```python
from build123d import *

# Parameters (mm, degrees)
F1_DEPTH  = 2
F2_DEPTH  = 25
F3_T      = -2
F4_W      = 8
F4_H      = 8
F5_DEPTH  = 25
F6_W      = 35
F6_H      = 11.5
F6_R      = 1.1
F7_DEPTH  = 30
F8_DEPTH  = 10
F9_W      = 25
F9_H      = 11.5
F10_DEPTH = 25
F11_DEPTH = 10


# Not quite as in the source:
# - a feature names something its author has since deleted; it is built from what else it names


with BuildPart() as f1:
    # F0 (on Top) → F1 (new body)
    with BuildSketch(Plane.XY):
        with BuildLine():
            Line((-20, -62.5), (20, -62.5))
            ThreePointArc((20, -62.5), (34.1421356237, -56.6421356237), (40, -42.5))
            Line((40, -42.5), (40, 42.5))
            ThreePointArc((40, 42.5), (34.1421356237, 56.6421356237), (20, 62.5))
            Line((20, 62.5), (-20, 62.5))
            ThreePointArc((-20, 62.5), (-34.1421356237, 56.6421356237), (-40, 42.5))
            Line((-40, 42.5), (-40, -42.5))
            ThreePointArc((-40, -42.5), (-34.1421356237, -56.6421356237), (-20, -62.5))
        make_face()
    extrude(amount=F1_DEPTH)

    # F0 (on Top) → F2 (join)
    with BuildSketch(Plane.XY):
        with BuildLine():
            Line((-20, -62.5), (20, -62.5))
            ThreePointArc((20, -62.5), (34.1421356237, -56.6421356237), (40, -42.5))
            Line((40, -42.5), (40, 42.5))
            ThreePointArc((40, 42.5), (34.1421356237, 56.6421356237), (20, 62.5))
            Line((20, 62.5), (-20, 62.5))
            ThreePointArc((-20, 62.5), (-34.1421356237, 56.6421356237), (-40, 42.5))
            Line((-40, 42.5), (-40, -42.5))
            ThreePointArc((-40, -42.5), (-34.1421356237, -56.6421356237), (-20, -62.5))
        make_face()
    extrude(amount=F2_DEPTH)

    # F3
    f3_openings = [f1.faces().sort_by_distance(p)[0] for p in [
        (0, 0, 25),
    ]]
    offset(amount=F3_T, openings=f3_openings)

    # F4 (on face) → F5 (cut)
    with BuildSketch(Plane.XY.offset(2)):
        with Locations((20, 0)):
            Rectangle(F4_W, F4_H)
        with Locations((-20, 0)):
            Rectangle(F4_W, F4_H)
    extrude(amount=-F5_DEPTH, mode=Mode.SUBTRACT)

    # F6 (on Front) → F7 (join)
    with BuildSketch(Plane.XZ):
        with Locations((0, 7.75)):
            Rectangle(F6_W, F6_H)
        with Locations((-13.8, 7.75)):
            Circle(F6_R, mode=Mode.SUBTRACT)
        with Locations((13.8, 7.75)):
            Circle(F6_R, mode=Mode.SUBTRACT)
    extrude(amount=-F7_DEPTH)

    # F8 (cut): a face of the model
    f8_faces = [f1.faces().sort_by_distance(p)[0] for p in [
        (0, 0, 7.75),
    ]]
    extrude(f8_faces, amount=-F8_DEPTH, mode=Mode.SUBTRACT)

    # F9 (on face) → F10 (cut)
    with BuildSketch(Plane.XZ.offset(-10)):
        with Locations((0, 7.75)):
            Rectangle(F9_W, F9_H)
    extrude(amount=-F10_DEPTH, mode=Mode.SUBTRACT)

    # F11 (cut): faces of the model
    f11_faces = [f1.faces().sort_by_distance(p)[0] for p in [
        (15.0849479566, 30, 7.75),
        (-15.0849479566, 30, 7.75),
    ]]
    extrude(f11_faces, amount=-F11_DEPTH, mode=Mode.SUBTRACT)


solid = f1.part
```
Here's how the part is built. I have some questions about the finished solid (model axes, mm). A direction names the side the tool comes from. Coordinates: 2 decimals unless noted, no trailing zeros. Loops run counter-clockwise (first coordinate to the right, second up) from the corner with the lowest first, then second, coordinate; pieces in that order, holes last. Notation, with made-up numbers: (77, -3) - (83, -3) arc R20 cw to (83, 5) - close; hole circle Ø8 at (19, 85). An arc over 180 degrees is marked (long way). Return JSON: item names as keys, results as strings. Group by question number.
Item 1: If we section it at A-A on z = 5: Write out the boundary of the cut face in (x, y).
Item 2: If we section it at C-C on z = 17: Write out the boundary of the cut face in (x, y).
Item 3: On a 3-axis mill with a long thin cutter (end or side, diameter ignored), from which of +Z, -Z, +X, -X, +Y, -Y can I reach the whole of each face in a straight line? I mean faces 5 (the face through (17.5, 15, 8)), 6 (the face through (34.297, 56.486, 12.325)). Say none if no direction works.
Item 4: Will these pins go through, and if not, where does the flat tip stop? P1, Ø4, axis at x = -12.5, y = 0, coming from the +Z side; P2, Ø10, axis at y = 49.5, z = 6, coming from the -X side; P3, Ø5, axis at x = -13, y = 16.5, coming from the +Z side; P4, Ø8, axis at x = 2, y = -42, coming from the -Z side.
Item 5: I need wall thicknesses on line 1 (Y direction, x = -21, z = 4.5); line 2 (X direction, y = -18, z = 12); line 3 (Z direction, x = -13.8, y = 13.5). Which ranges of each line are inside material? Lowest first, please. Write a range as from..to.
Item 6: If we section it at B-B on y = 6: Write out the boundary of the cut face in (x, z).
Item 7: We'd pull the mould along X, two halves only. Please class faces 1 (the face through (-33.986, 56.797, 12.325)), 2 (the face through (38, -1, 13)), 3 (the face through (-15, 15, 13.5)), 4 (the face through (33.986, -56.797, 12.325)): +X half, -X half, draft (parallel to the pull), parting line (faces both ways), or undercut.
Item 8: If we section it at D-D on x = -22: Write out the boundary of the cut face in (y, z), and give its area (3 significant figures).
Calculated:
{
 "1": {"outline": "(-40, -42.5) arc R20 ccw to (-20, -62.5) - (20, -62.5) arc R20 ccw to (40, -42.5) - (40, 42.5) arc R20 ccw to (20, 62.5) - (-20, 62.5) arc R20 ccw to (-40, 42.5) - close; (-17.5, 10) - (-12.5, 10) - (-12.5, 20) - (-17.5, 20) - close; (12.5, 10) - (17.5, 10) - (17.5, 20) - (12.5, 20) - close; hole (-38, -42.5) arc R18 ccw to (-20, -60.5) - (20, -60.5) arc R18 ccw to (38, -42.5) - (38, 42.5) arc R18 ccw to (20, 60.5) - (-20, 60.5) arc R18 ccw to (-38, 42.5) - close"},
 "2": {"outline": "(-40, -42.5) arc R20 ccw to (-20, -62.5) - (20, -62.5) arc R20 ccw to (40, -42.5) - (40, 42.5) arc R20 ccw to (20, 62.5) - (-20, 62.5) arc R20 ccw to (-40, 42.5) - close; hole (-38, -42.5) arc R18 ccw to (-20, -60.5) - (20, -60.5) arc R18 ccw to (38, -42.5) - (38, 42.5) arc R18 ccw to (20, 60.5) - (-20, 60.5) arc R18 ccw to (-38, 42.5) - close"},
 "3": {"face 5": "+Z", "face 6": "+Z, -Z, +X, +Y"},
 "4": {"P1": "stops at z = 2", "P2": "stops at x = -39.9", "P3": "stops at z = 13.5", "P4": "stops at z = 0"},
 "5": {"line 1": "y = -62.47..-60.47, 60.47..62.47", "line 2": "x = -40..-38, 38..40", "line 3": "z = 0..6.65, 8.85..13.5"},
 "6": {"outline": "(-40, 0) - (40, 0) - (40, 25) - (38, 25) - (38, 2) - (-38, 2) - (-38, 25) - (-40, 25) - close"},
 "7": {"face 1": "-X half", "face 2": "undercut", "face 3": "undercut", "face 4": "+X half"},
 "8": {"outline": "(-62.4, 0) - (-4, 0) - (-4, 2) - (-60.39, 2) - (-60.39, 25) - (-62.4, 25) - close; (4, 0) - (62.4, 0) - (62.4, 25) - (60.39, 25) - (60.39, 2) - (4, 2) - close", "area": "326 mm^2"}
}
